The listing builds one solid part. Answer for the finished solid, in the listing's coordinates (mm). A direction names the side the tool comes from. Give positions to 0.01 mm unless a question says otherwise; leave off trailing zeros. Order: outer loops, then holes, each group sorted by start corner. A loop starts at its lowest first (then second) coordinate and runs counter-clockwise, first axis right, second up. Notation, with made-up numbers: (32, -24.5) - (49, -24.5) arc R24 ccw to (49, -6.5) - close; hole circle Ø4 at (-22, -36). An arc over 180 degrees is marked (long way). Answer as CSV lines item,"result". Start each with the question number.
1. Consider line 1 along Z through (x, y) = (0, -34.5); line 2 along Z through (x, y) = (0, -3.25); line 3 along X through (y, z) = (-49.5, -4). Determine where each line is inside the solid, lowest interval first. Write a range as [from, to].
2. Section A-A on x = 0 is taken. Give the vertices of the cut face in (y, z), and give its area (4 significant figures).
3. Section D-D on z = -6.75 is taken. Give the vertices of the cut face in (x, y), and give its area (3 significant figures).
4. Section C-C on y = -32 is taken. Give the vertices of the cut face in (x, z), and give its area (3 significant figures).
5. Which of the six approach directions +Z, -Z, +X, -X, +Y, -Y give full straight-line access (tool end or side, diameter ignored) to faces 1 (the cylindrical face through (-1.009, -42.955, 7.684)), 2 (the flat face through (0, 0, -6))?
6. Determine the mould class of faces 3 (the cylindrical face through (-1.172, -36.975, 8.923)), 4 (the cylindrical face through (5.794, -4.93, 0.255)), 5 (the flat face through (4, -75, 7)) for opening direction Z: +Z half, -Z half, draft (parallel to the pull), parting line (faces both ways), or undercut.
7. Flat-ended cylindrical pins translate along their axes: pin 1 (1.5 mm diameter, centred on y = -45, z = 1, fed in from +X); pin 2 (6 mm diameter, centred on x = -5, y = -53, fed in from +Z); pin 3 (3 mm diameter, centred on x = 3, y = -12.5, fed in from -Z). Find the tip coordinate at first contact, or state that the pin passes through.
8. Section B-B on z = 0 is taken. Give the vertices of the cut face in (x, y).
from build123d import *

# Parameters (mm, degrees)
F0_R     = 9
F1_DEPTH = 75
F2_R     = 7.75
F3_DEPTH = 65
F4_R     = 5.8
F5_DEPTH = 75.001


with BuildPart() as f1:
    # F0 (on Front) → F1 (new body)
    with BuildSketch(Plane.XZ):
        Circle(F0_R)
    extrude(amount=F1_DEPTH)

    # F2 (on face) → F3 (cut)
    with BuildSketch(Plane.XZ.offset(75)):
        Circle(F2_R)
    extrude(amount=-F3_DEPTH, mode=Mode.SUBTRACT)

    # F4 (on face) → F5 (cut, through all)
    with BuildSketch(Plane(origin=(0, 0, 0), x_dir=(-1, 0, 0), z_dir=(0, 1, 0))):
        Circle(F4_R)
    extrude(amount=-F5_DEPTH, mode=Mode.SUBTRACT)


solid = f1.part
Checks:
1,line 1,"z = [-9, -7.75], [7.75, 9]"
1,line 2,"z = [-9, -5.8], [5.8, 9]"
1,line 3,"x = [-8.06, -6.64], [6.64, 8.06]"
2,outline,"(-75, -9) - (0, -9) - (0, -5.8) - (-10, -5.8) - (-10, -7.75) - (-75, -7.75) - close; (-75, 7.75) - (-10, 7.75) - (-10, 5.8) - (0, 5.8) - (0, 9) - (-75, 9) - close"
2,area,"226.5 mm²"
3,outline,"(-5.95, -75) - (-3.81, -75) - (-3.81, -10) - (3.81, -10) - (3.81, -75) - (5.95, -75) - (5.95, 0) - (-5.95, 0) - close"
3,area,"398 mm²"
4,outline,"circle Ø18 at (0, 0); hole circle Ø15.5 at (0, 0)"
4,area,"65.8 mm²"
5,face 1,"-Y"
5,face 2,"+Z, -Z, +X, -X, +Y"
6,face 3,"parting line"
6,face 4,"undercut"
6,face 5,"draft"
7,pin 1,"stops at x = 9"
7,pin 2,"stops at z = 8.77"
7,pin 3,"stops at z = -8.87"
8,outline,"(-9, -75) - (-7.75, -75) - (-7.75, -10) - (-5.8, -10) - (-5.8, 0) - (-9, 0) - close; (5.8, -10) - (7.75, -10) - (7.75, -75) - (9, -75) - (9, 0) - (5.8, 0) - close"
